Autodesk Inventor part; units mm, degrees
ref_plane "YZ Plane" through (0, 0, 0) normal (1, 0, 0) x (0, 1, 0)
ref_plane "XZ Plane" through (0, 0, 0) normal (0, 1, 0) x (-1, 0, 0)
ref_plane "XY Plane" through (0, 0, 0) normal (0, 0, 1) x (1, 0, 0)
sketch "Esboço1" plane through (0, 0, 0) normal (0, 1, 0) x (-1, 0, 0)
  line L0 (131.25, 130.95) -> (-131.25, 130.95)
  line L1 (-131.25, 130.95) -> (-131.25, -130.95)
  line L2 (-131.25, -130.95) -> (131.25, -130.95)
  line L3 (131.25, -130.95) -> (131.25, 130.95)
  line L4 (131.25, 130.95) -> (-131.25, -130.95) construction
  line L5 (-131.25, 130.95) -> (131.25, -130.95) construction
  line L6 (-131.25, -110.25) -> (131.25, -110.25)
  line L7 (131.25, 110.25) -> (-131.25, 110.25)
  line L8 (100.15, -130.95) -> (100.15, 130.95)
  line L9 (-100.15, 130.95) -> (-100.15, -130.95)
  line L10 (131.25, 100.25) -> (-131.25, 100.25)
  line L11 (-131.25, -100.25) -> (131.25, -100.25)
  point P0 (0, 0)
  point P1 (-100.15, -100.25)
  point P2 (100.15, -100.25)
  point P3 (100.15, 100.25)
  point P4 (-100.15, 100.25)
  dimension "d0" = 262.5
  dimension "d1" = 261.9
  dimension "d2" = 20.7
  dimension "d3" = 20.7
  dimension "d4" = 31.1
  dimension "d5" = 31.1
  dimension "d6" = 10
  dimension "d7" = 10
extrude "Extrusão1" add sketch "Esboço1" along normal blind 68.8
extrude "Extrusão2" cut sketch "Esboço1" along normal blind 68.8 contours L8 L11 L9 L10
sketch "Esboço2" plane through (0, 68.8, 0) normal (0, 1, 0) x (1, 0, 0)
  line L0 (100.15, 100.25) -> (-100.15, 100.25)
  line L1 (-100.15, -100.25) -> (-100.15, 100.25)
  line L2 (-100.15, 100.25) -> (-100.15, -100.25)
  line L3 (-100.15, 100.25) -> (-100.15, -100.25)
  line L4 (-100.15, -100.25) -> (-100.15, 100.25)
  line L5 (-131.25, 130.95) -> (-131.25, -130.95)
  line L6 (-131.25, 130.95) -> (-131.25, -130.95)
  line L7 (-131.25, 130.95) -> (-131.25, -130.95)
  line L8 (-131.25, 130.95) -> (-131.25, -130.95)
  line L9 (131.25, 130.95) -> (-131.25, 130.95)
  line L10 (-100.15, -100.25) -> (100.15, -100.25)
  line L11 (-131.25, -130.95) -> (131.25, -130.95)
  line L12 (100.15, 100.25) -> (-100.15, 100.25)
  line L13 (-100.15, 100.25) -> (-100.15, -100.25)
  line L14 (-100.15, -100.25) -> (100.15, -100.25)
  line L15 (100.15, -100.25) -> (100.15, 100.25)
  line L16 (-131.25, -130.95) -> (131.25, -130.95)
  line L17 (-131.25, 130.95) -> (-131.25, -130.95)
  line L18 (131.25, 130.95) -> (-131.25, 130.95)
  line L19 (131.25, -130.95) -> (131.25, 130.95)
  line L20 (131.25, -130.95) -> (131.25, 130.95)
  line L21 (100.15, -100.25) -> (100.15, 100.25)
  line L22 (-131.25, -130.95) -> (131.25, -130.95)
  line L23 (-131.25, -110.25) -> (131.25, -110.25)
  line L24 (-131.25, -100.25) -> (131.25, -100.25)
  line L25 (131.25, -130.95) -> (131.25, 130.95)
  line L26 (100.15, -130.95) -> (100.15, 130.95)
  line L27 (-100.15, 130.95) -> (-100.15, -130.95)
  line L28 (-131.25, -130.95) -> (131.25, 130.95) construction
  line L29 (-131.25, 130.95) -> (-131.25, -130.95)
  line L30 (131.25, -130.95) -> (-131.25, 130.95) construction
  line L31 (131.25, 100.25) -> (-131.25, 100.25)
  line L32 (131.25, 110.25) -> (-131.25, 110.25)
  line L33 (131.25, 130.95) -> (-131.25, 130.95)
  point P0 (0, 0)
  point P1 (0, 0)
  point P2 (-100.15, -110.25)
  point P3 (100.15, -110.25)
  point P4 (100.15, 110.25)
  point P5 (-100.15, 110.25)
extrude "Extrusão3" cut sketch "Esboço2" against normal blind 10 contours L0 L27 L32 L26 | L26 L23 L27 L10
properties part number "Melgueira-Sobreninho"
Source: CAD feature listing. Evaluate the final solid. Frame: model axes, mm. A direction names the side the tool comes from. Give positions to 0.01 mm unless a question says otherwise; leave off trailing zeros. Loops run counter-clockwise (first coordinate to the right, second up) from the corner with the lowest first, then second, coordinate; pieces in that order, holes last. Notation, with made-up numbers: (11.25, -8) -> (55.25, -8) arc R30 ccw to (55.25, 22) -> close; hole circle Ø7 at (36, -38). An arc over 180 degrees is marked (long way). Use a Markdown table: item, result. Add a question column.
1) Section query B-B, the plane z = 53. Return the cut outline in (x, y), then the cut area to 3 significant figures.
2) Section query A-A, the plane x = -76.5. Return the cut outline in (y, z), then the cut area to 3 significant figures.
3) Section query C-C, the plane y = 51.5. Return the cut outline in (x, z), then the cut area to 3 significant figures.
4) Reachability of faces 1 (the face through (1, 29, -100.25)), 2 (the face through (-1, 58.8, 105)), 3 (the face through (131.25, 34, 2)) from +Z, -Z, +X, -X, +Y, -Y: full face, straight path, thin tool, end or side. Return the list, or none.
5) Pull-direction query (Z, two-part tool) for faces 4 (the face through (-131.25, 34, -2)), 5 (the face through (-2, 34, 130.95)), 6 (the face through (2, 34, -130.95)), 7 (the face through (1, 64, -110.25)); classes: +Z half, -Z half, draft (parallel to the pull), parting line (faces both ways), or undercut.
6) Line query: line 1 along X through (y, z) = (21, 29.5); line 2 along Z through (x, y) = (-34, 47.5). Output: solid intervals per line, ascending. Write a range as [from, to].
7) First-contact query: pin 1 (3 mm diameter, centred on x = -5, z = 106, fed in from +Y); pin 2 (12 mm diameter, centred on x = -96.5, z = 94.5, fed in from +Y); pin 3 (6 mm diameter, centred on x = 88.5, z = 95.5, fed in from +Y) (3 decimals). Flat tips, straight axial feed; report the tip coordinate or a pass-through.
Numbers:
| question | item | result |
|---|---|---|
| 1 | outline | (-131.25, 0) -> (-100.15, 0) -> (-100.15, 68.8) -> (-131.25, 68.8) -> close; (100.15, 0) -> (131.25, 0) -> (131.25, 68.8) -> (100.15, 68.8) -> close |
| 1 | area | 4,280 mm2 |
| 2 | outline | (0, -130.95) -> (68.8, -130.95) -> (68.8, -110.25) -> (58.8, -110.25) -> (58.8, -100.25) -> (0, -100.25) -> close; (0, 100.25) -> (58.8, 100.25) -> (58.8, 110.25) -> (68.8, 110.25) -> (68.8, 130.95) -> (0, 130.95) -> close |
| 2 | area | 4,020 mm2 |
| 3 | outline | (-131.25, -130.95) -> (131.25, -130.95) -> (131.25, 130.95) -> (-131.25, 130.95) -> close; hole (-100.15, -100.25) -> (100.15, -100.25) -> (100.15, 100.25) -> (-100.15, 100.25) -> close |
| 3 | area | 28,600 mm2 |
| 4 | face 1 | +Y, -Y |
| 4 | face 2 | +Y |
| 4 | face 3 | +Z, -Z, +X, +Y, -Y |
| 5 | face 4 | draft |
| 5 | face 5 | +Z half |
| 5 | face 6 | -Z half |
| 5 | face 7 | undercut |
| 6 | line 1 | x = [-131.25, -100.15], [100.15, 131.25] |
| 6 | line 2 | z = [-130.95, -100.25], [100.25, 130.95] |
| 7 | pin 1 | stops at y = 58.8 |
| 7 | pin 2 | stops at y = 68.8 |
| 7 | pin 3 | passes through |
